Job drawing, mm, ordinate dimensions from the low corner. One solid piece. A direction names the side the tool comes from. Give positions to 0.01 mm unless a question says otherwise; leave off trailing zeros. Write each loop counter-clockwise with the first axis right and the second up, starting at its lowest first coordinate (ties: lowest second). Pieces come first, ordered by that corner, then holes. Notation, with made-up numbers: M -27,36 L -16,36 A19 cw -16,65 Z; hole C 26.25,-30.5 d9. An arc over 180 degrees is marked long. Use CSV: the item, a comma, the result in double quotes. Start each with the question number.
Item 1: Which spindle directions (+Z, -Z, +X, -X, +Y, -Y) get a long thin tool onto all of the face, cutting with end or side? Do the marked faces 1 and 2. Say none if no direction does.
Item 2: Cut at D-D (z = 4.5). List the corners of the cut face in (x, y) (1 decimal).
Item 3: Cut at A-A (x = 14.25). List the corners of the cut face in (y, z), then the cut area to 3 significant figures.
Item 4: Pin check, flat tip, straight feed: pin 1 (0.9 mm diameter, centred on y = 12.5, z = 5.5, fed in from +X) (1 decimal). Stop position of the tip, or through.
Item 5: Mould opens along Y. For the marked faces 3, 4 and 5 say: released by +Y, released by -Y, zero draft, split by the parting line, or undercut.
Item 6: Drill centre lines: line 1 (Y direction, x = 13, z = 10); line 2 (Y direction, x = 13.5, z = 12.5); line 3 (X direction, y = 23.75, z = 11.5). Where is each one in solid material? Low to high. Write a range as [from, to].
Item 7: Cut at C-C (y = 7). List the corners of the cut face in (x, z).
Item 8: Cut at B-B (z = 9.25). Count the separate pieces of the cut face and the enclosed holes in it, then the cut area to 3 significant figures.
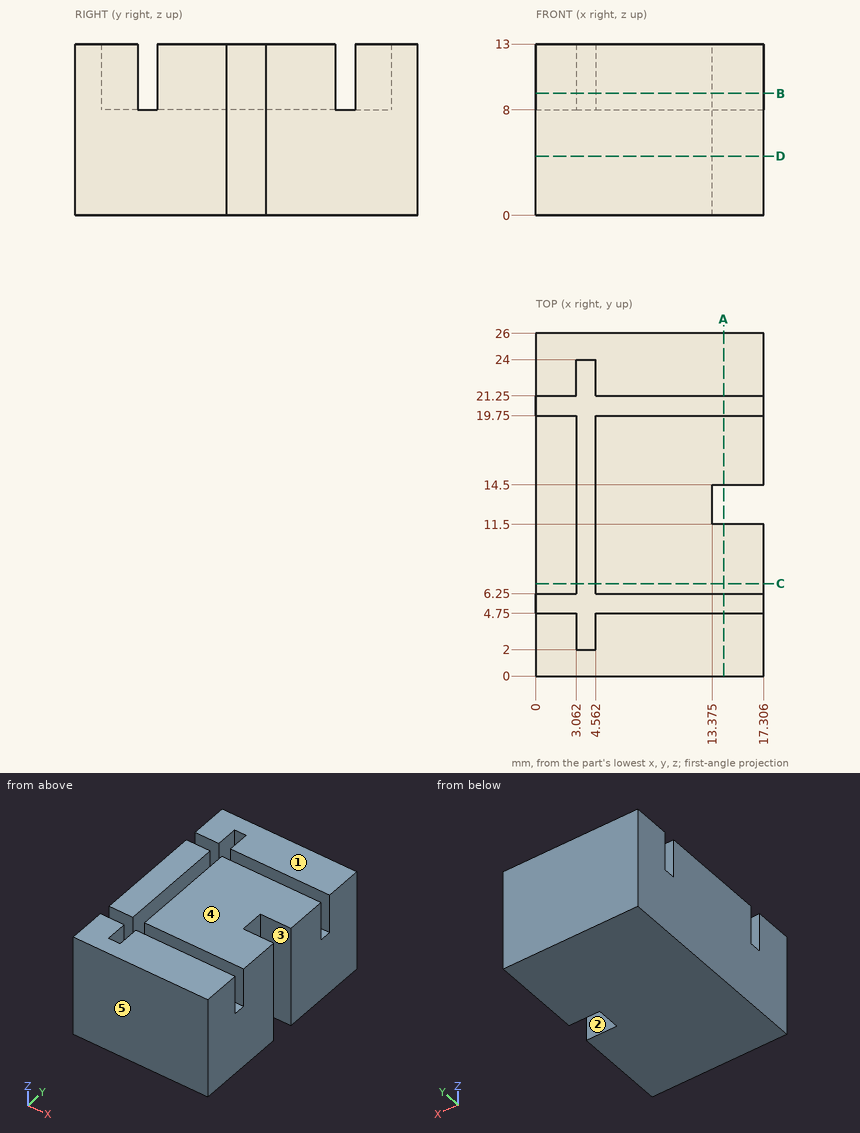
Worked answers:
1,face 1,"+Z, +X, -X, +Y, -Y"
1,face 2,"+Z, -Z, +X"
2,outline,"M 0,0 L 17.3,0 L 17.3,11.5 L 13.4,11.5 L 13.4,14.5 L 17.3,14.5 L 17.3,26 L 0,26 Z"
3,outline,"M 0,0 L 11.5,0 L 11.5,13 L 6.25,13 L 6.25,8 L 4.75,8 L 4.75,13 L 0,13 Z; M 14.5,0 L 26,0 L 26,13 L 21.25,13 L 21.25,8 L 19.75,8 L 19.75,13 L 14.5,13 Z"
3,area,"284 mm^2"
4,pin 1,"stops at x = 13.4"
5,face 3,"undercut"
5,face 4,"zero draft"
5,face 5,"released by -Y"
6,line 1,"y = [0, 4.75], [6.25, 19.75], [21.25, 26]"
6,line 2,"y = [0, 4.75], [6.25, 11.5], [14.5, 19.75], [21.25, 26]"
6,line 3,"x = [0, 3.06], [4.56, 17.31]"
7,outline,"M 0,0 L 17.31,0 L 17.31,13 L 4.56,13 L 4.56,8 L 3.06,8 L 3.06,13 L 0,13 Z"
8,separate pieces,"4"
8,enclosed holes,"0"
8,area,"358 mm^2"
